Input: part model. Units: mm. Frame: model coordinates. A direction names the side the tool comes from. Round coordinates to 2 decimals unless told otherwise and drop trailing zeros. Loops run counter-clockwise (first coordinate to the right, second up) from the corner with the lowest first, then second, coordinate; pieces in that order, holes last. Notation, with made-up numbers: (85, -36.75) -> (121, -36.75) arc R21 ccw to (121, -7.75) -> close; hole circle Ø2 at (-10, 50). An arc over 180 degrees is marked (long way). Answer as a JSON object with one key per item and string values. Group by question number.
Item 1: Section query A-A on y = 0. Return loops of the section in (x, z), and give its area (3 significant figures).
Item 2: Set-up query: faces 1 (the flat face through (-8, -0.1, 0.5)), 2 (the flat face through (-2, 5, 1.5)), 3 (the cylindrical face through (0.867, -3.905, 1.232)). Return all of +Z, -Z, +X, -X, +Y, -Y with unobstructed straight access to the full face (end or side cutting, diameter ignored); none if empty.
Item 3: Pin query (flat end, axial travel): pin 1 (1.8 mm diameter, centred on x = 5.5, y = -5.5, fed in from -Z); pin 2 (5 mm diameter, centred on x = 1.5, y = 0.5, fed in from -Z); pin 3 (2.5 mm diameter, centred on x = 0.5, y = -1, fed in from -Z); pin 4 (3 mm diameter, centred on x = -5.5, y = 5.5, fed in from +Z). Return the tip coordinate at first contact, or that it passes through.
Item 4: Section query B-B on x = 5.5. Return loops of the section in (y, z), and give its area (3 significant figures).
Item 5: Draft query along X for faces 4 (the cylindrical face through (-7.4, -7.43, 0.49)), 5 (the flat face through (0.1, -8, 0.5)), 6 (the cylindrical face through (-1.08, 4.88, 3.72)), 7 (the cylindrical face through (6.237, -4.824, 0.74)). Return one class per face: released by +X, released by -X, zero draft, split by the parting line, or undercut.
Item 6: Material intervals for line 1 (Y direction, x = 0, z = 0.8); line 2 (Z direction, x = -6, y = 2.5); line 3 (Y direction, x = 5.5, z = 1.25), sorted ascending. Write a range as [from, to].
Autodesk Inventor part; units mm, degrees
ref_plane "YZ Plane" through (0, 0, 0) normal (1, 0, 0) x (0, 1, 0)
ref_plane "XZ Plane" through (0, 0, 0) normal (0, 1, 0) x (-1, 0, 0)
ref_plane "XY Plane" through (0, 0, 0) normal (0, 0, 1) x (1, 0, 0)
sketch "Sketch1" plane through (0, 0, 0) normal (0, 0, 1) x (1, 0, 0)
  line L0 (-6, 8) -> (6, 8)
  line L1 (8, 6) -> (8, -6)
  line L2 (6, -8) -> (-6, -8)
  line L3 (-8, -6) -> (-8, 6)
  line L4 (-8, 8) -> (8, -8) construction
  line L5 (8, 8) -> (-8, -8) construction
  arc A0 (-6, 8) -> (-8, 6) centre (-6, 6) ccw
  arc A1 (-8, -6) -> (-6, -8) centre (-6, -6) ccw
  arc A2 (8, 6) -> (6, 8) centre (6, 6) ccw
  arc A3 (6, -8) -> (8, -6) centre (6, -6) ccw
  point P0 (0, 0)
  dimension "d0" = 16
  dimension "d1" = 16
  dimension "d2" = 2
extrude "Extrusion1" add sketch "Sketch1" along normal blind 1.5
sketch "Sketch2" plane through (0, 0, 1.5) normal (0, 0, 1) x (1, 0, 0)
  circle A0 centre (0, 0) radius 5
  dimension "d5" = 10
extrude "Extrusion2" add sketch "Sketch2" along normal blind 5
fillet "Fillet1" radius 0.5 9 edges at (-5, 0, 6.5) (-7.4142, 7.4142, 1.5) (-8, 0, 1.5) (-7.4142, -7.4142, 1.5) (0, -8, 1.5) (7.4142, -7.4142, 1.5) (8, 0, 1.5) (7.4142, 7.4142, 1.5) (0, 8, 1.5)
sketch "Sketch3" plane through (0, 0, 6.5) normal (0, 0, 1) x (1, 0, 0)
  circle A0 centre (0, 0) radius 4.5
  circle A1 centre (0, 0) radius 1.5
  dimension "d9" = 3
extrude "Extrusion3" cut sketch "Sketch3" against normal through all contours A1
sketch "Sketch4" plane through (0, 0, 0) normal (0, 0, -1) x (-1, 0, 0)
  circle A0 centre (0, 0) radius 1.5
  circle A1 centre (0, 0) radius 4
  dimension "d12" = 8
extrude "Extrusion4" cut sketch "Sketch4" against normal blind 2.5
sketch "Sketch5" plane through (0, 0, 0) normal (0, 0, -1) x (-1, 0, 0)
  line L0 (6, -8) -> (-6, -8)
  line L1 (8, 6) -> (8, -6)
  line L2 (-8, -6) -> (-8, 6)
  circle A0 centre (-5.5, 5.5) radius 1
  circle A1 centre (5.5, 5.5) radius 1
  circle A2 centre (5.5, -5.5) radius 1
  circle A3 centre (-5.5, -5.5) radius 1
  dimension "d15" = 2.5
  dimension "d16" = 2.5
  dimension "d17" = 11
  dimension "d18" = 2
  dimension "d19" = 2.5
extrude "Extrusion5" cut sketch "Sketch5" against normal through all
properties part number "12B VALVE BONNET" material "Steel AISI 1020 107 HR"
Solved:
{
 "1": {"outline": "(-8, 0) -> (-4, 0) -> (-4, 2.5) -> (-1.5, 2.5) -> (-1.5, 6.5) -> (-4.5, 6.5) arc R0.5 ccw to (-5, 6) -> (-5, 1.5) -> (-7.5, 1.5) arc R0.5 ccw to (-8, 1) -> close; (1.5, 2.5) -> (4, 2.5) -> (4, 0) -> (8, 0) -> (8, 1) arc R0.5 ccw to (7.5, 1.5) -> (5, 1.5) -> (5, 6) arc R0.5 ccw to (4.5, 6.5) -> (1.5, 6.5) -> close", "area": "41.8 mm²"},
 "2": {"face 1": "+Z, -Z, -X, +Y, -Y", "face 2": "+Z", "face 3": "-Z"},
 "3": {"pin 1": "through", "pin 2": "z = 0", "pin 3": "z = 2.5", "pin 4": "z = 1.5"},
 "4": {"outline": "(-8, 0) -> (-6.5, 0) -> (-6.5, 1.5) -> (-7.5, 1.5) arc R0.5 ccw to (-8, 1) -> close; (-4.5, 0) -> (4.5, 0) -> (4.5, 1.5) -> (-4.5, 1.5) -> close; (6.5, 0) -> (8, 0) -> (8, 1) arc R0.5 ccw to (7.5, 1.5) -> (6.5, 1.5) -> close", "area": "17.9 mm²"},
 "5": {"face 4": "released by -X", "face 5": "zero draft", "face 6": "split by the parting line", "face 7": "undercut"},
 "6": {"line 1": "[-8, -4], [4, 8]", "line 2": "[0, 1.5]", "line 3": "[-7.93, -6.5], [-4.5, 4.5], [6.5, 7.93]"}
}
